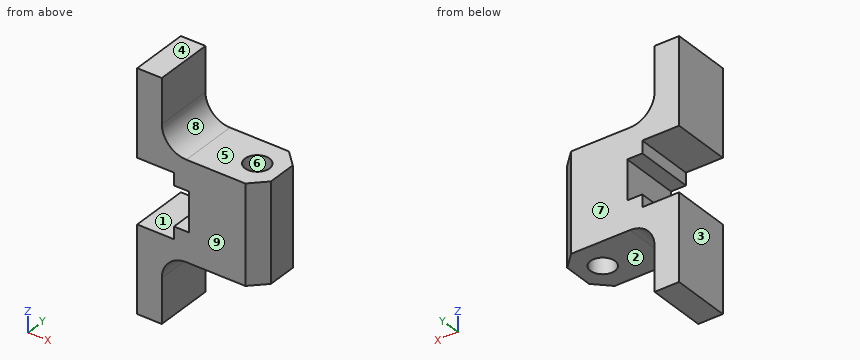
```python
from build123d import *

# Parameters (mm, degrees)
SKETCH_1_W          = 20
SKETCH_1_H          = 12
EXTRUDE_1_DEPTH     = 25
SKETCH_5_R          = 2.5
CUT_EXTRUDE_2_DEPTH = 57.563315968
SKETCH_6_W          = 14
SKETCH_6_H          = 12
EXTRUDE_2_DEPTH     = 5
CHAMFER_1_SIZE      = 3
CUT_EXTRUDE_3_DEPTH = 44.874821937
FILLET_1_R          = 5


with BuildPart() as part:
    # Эскиз1 → Вытянуть1 (new body)
    with BuildSketch(Plane(origin=(0, 0, 0), x_dir=(0, 0, -1), z_dir=(1, 0, 0))):
        with Locations((-10, -40.630555576)):
            Rectangle(SKETCH_1_W, SKETCH_1_H)
    extrude(amount=EXTRUDE_1_DEPTH)

    # Эскиз5 → Вырез-Вытянуть2 (cut, through all)
    with BuildSketch(Plane.XY.offset(20)):
        with Locations((20, -40.630555576)):
            Circle(SKETCH_5_R)
    extrude(amount=-CUT_EXTRUDE_2_DEPTH, mode=Mode.SUBTRACT)

    # Эскиз6 → Вытянуть2 (add)
    with BuildSketch(Plane.ZY):
        with Locations((27, -40.630555576)):
            Rectangle(SKETCH_6_W, SKETCH_6_H)
        with Locations((-7, -40.630555576)):
            Rectangle(SKETCH_6_W, SKETCH_6_H)
    extrude(amount=-EXTRUDE_2_DEPTH)

    # Фаска1
    chamfer_1_edges = [part.edges().sort_by_distance(p)[0] for p in [
        (25, -46.630555576, 10),
        (25, -34.630555576, 10),
    ]]
    chamfer(chamfer_1_edges, length=CHAMFER_1_SIZE)

    # Эскиз8 → Вытянуть3 (cut, through all)
    with BuildSketch(Plane(origin=(0, -34.630555576, 0), x_dir=(1, 0, 0), z_dir=(0, 1, 0))):
        Polygon((-15.5, -3.5), (7.5, -3.5), (7.5, -6), (10.541246576, -6), (10.541246576, -14), (7.5, -14), (7.5, -16.5), (-15.5, -16.5), align=None)
    extrude(amount=-CUT_EXTRUDE_3_DEPTH, mode=Mode.SUBTRACT)

    # Скругление1
    fillet_1_edges = [part.edges().sort_by_distance(p)[0] for p in [
        (5, -40.630555576, 0),
        (5, -40.630555576, 20),
    ]]
    fillet(fillet_1_edges, radius=FILLET_1_R)


solid = part.part
```
CAD build for the part. Positions are in the model's coordinates, mm. Face numbers are marked on the shaded views. A direction names the side the tool comes from. Give positions to 0.01 mm unless a question says otherwise; leave off trailing zeros. Order: outer loops, then holes, each group sorted by start corner. A loop starts at its lowest first (then second) coordinate and runs counter-clockwise, first axis right, second up.
(1) Saw through at B-B, the plane y = -40. Give the cut face in (x, z), then the cut area to 3 significant figures.
(2) Mould opens along Y. For the marked faces 6, 7, 8 and 9 say: released by +Y, released by -Y, zero draft, split by the parting line, or undercut.
(3) Drill centre lines: L1, parallel to Z at x = 10, y = -37.5; L2, parallel to Y at x = 20, z = 10.75; L3, parallel to Z at x = 3, y = -41.25. Where is each one in solid material? Low to high.
(4) Saw through at D-D, the plane y = -42.25. Give the cut face in (x, z), then the cut area to 3 significant figures.
(5) Saw through at C-C, the plane z = 3. Give the cut face in (x, y), then the cut area to 3 significant figures.
(6) Flat gauge pins, fed straight in: pin 1 (7 mm diameter, centred on y = -40.5, z = -11, fed in from +X); pin 2 (3 mm diameter, centred on y = -42.5, z = 4.5, fed in from -X); pin 3 (6 mm diameter, centred on x = 14, y = -43.5, fed in from -Z); pin 4 (6 mm diameter, centred on x = 18, y = -41.5, fed in from +Z). Where does each tip first touch, or does it go through?
(7) Tool access for the marked faces 1, 2, 3, 4 and 5: list every direction of +Z, -Z, +X, -X, +Y, -Y with a clear straight run to the whole face (end or side of a thin tool).
(8) Saw through at A-A, the plane x = 20. Give the cut face in (y, z), then the cut area to 3 significant figures.
Results found:
1. outline: (0, -14) - (5, -14) - (5, -5) arc R5 cw to (10, 0) - (17.58, 0) - (17.58, 20) - (10, 20) arc R5 cw to (5, 25) - (5, 34) - (0, 34) - (0, 16.5) - (7.5, 16.5) - (7.5, 14) - (10.54, 14) - (10.54, 6) - (7.5, 6) - (7.5, 3.5) - (0, 3.5) - close; (22.42, 0) - (25, 0) - (25, 20) - (22.42, 20) - close
1. area: 432 mm2
2. face 6: undercut
2. face 7: released by +Y
2. face 8: zero draft
2. face 9: released by -Y
3. L1: z = 0 to 6, 14 to 20
3. L2: y = -46.63 to -43.13, -38.13 to -34.63
3. L3: z = -14 to 3.5, 16.5 to 34
4. outline: (0, -14) - (5, -14) - (5, -5) arc R5 cw to (10, 0) - (18.1, 0) - (18.1, 20) - (10, 20) arc R5 cw to (5, 25) - (5, 34) - (0, 34) - (0, 16.5) - (7.5, 16.5) - (7.5, 14) - (10.54, 14) - (10.54, 6) - (7.5, 6) - (7.5, 3.5) - (0, 3.5) - close; (21.9, 0) - (25, 0) - (25, 20) - (21.9, 20) - close
4. area: 453 mm2
5. outline: (0, -46.63) - (22, -46.63) - (25, -43.63) - (25, -37.63) - (22, -34.63) - (0, -34.63) - close; hole circle Ø5 at (20, -40.63)
5. area: 271 mm2
6. pin 1: stops at x = 5
6. pin 2: stops at x = 0
6. pin 3: stops at z = 0
6. pin 4: stops at z = 20
7. face 1: -X, +Y, -Y
7. face 2: -Z, +X, +Y, -Y
7. face 3: +Z, -Z, -X, +Y, -Y
7. face 4: +Z, +X, -X, +Y, -Y
7. face 5: +Z, +X, +Y, -Y
8. outline: (-46.63, 0) - (-43.13, 0) - (-43.13, 20) - (-46.63, 20) - close; (-38.13, 0) - (-34.63, 0) - (-34.63, 20) - (-38.13, 20) - close
8. area: 140 mm2
